Job drawing, mm, ordinate dimensions from the low corner. One solid piece. A direction names the side the tool comes from. Coordinates: 2 decimals unless noted, no trailing zeros. Order: outer loops, then holes, each group sorted by start corner. A loop starts at its lowest first (then second) coordinate and runs counter-clockwise, first axis right, second up. Notation, with made-up numbers: (82, 22) - (135, 22) arc R18 ccw to (135, 42) - close; hole circle Ø10 at (-24.75, 49.5). An arc over 180 degrees is marked (long way). Return JSON: item names as keys, results as strings.
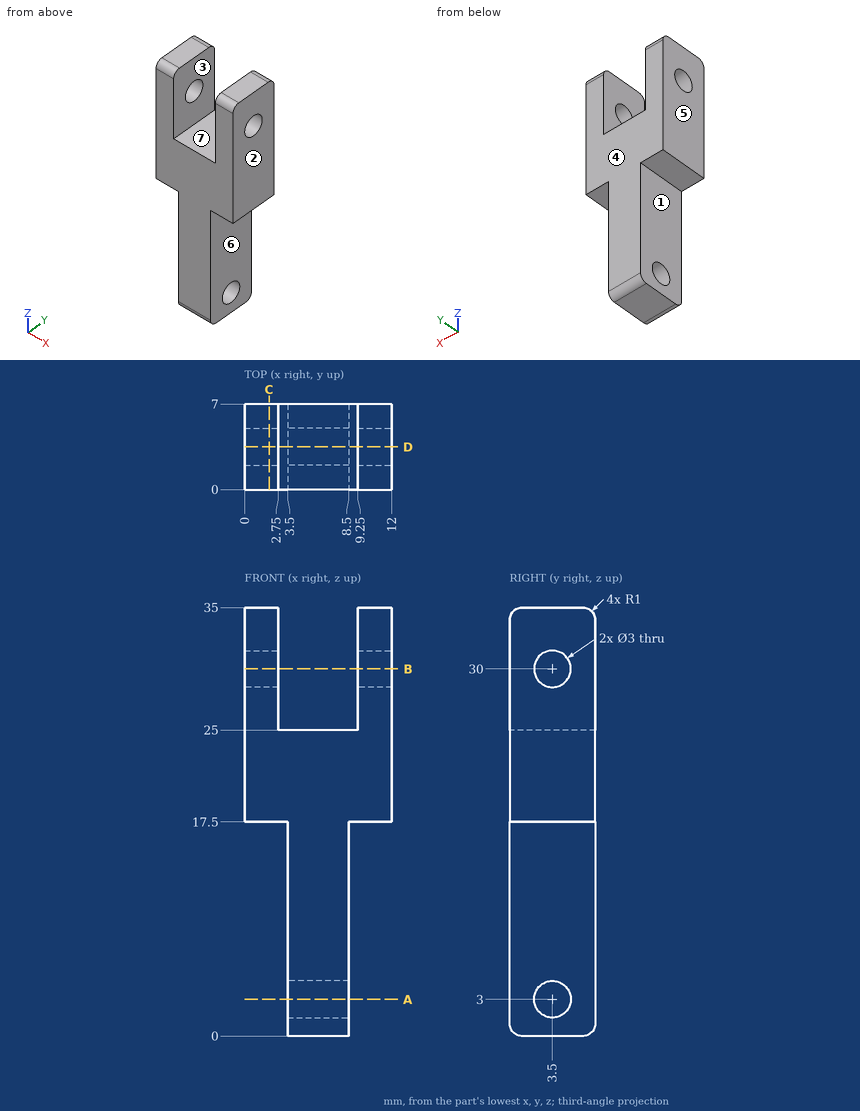
1. Cut at B-B on z = 30. Give the cut face in (x, y).
Check values:
{"outline": "(0, 0) - (2.75, 0) - (2.75, 2) - (0, 2) - close; (0, 5) - (2.75, 5) - (2.75, 7) - (0, 7) - close; (9.25, 0) - (12, 0) - (12, 2) - (9.25, 2) - close; (9.25, 5) - (12, 5) - (12, 7) - (9.25, 7) - close"}
2. Mould opens along X. For the marked faces 4, 5, 6 and 7 say: pulls with the +X half, pulls with the -X half, needs draft (parallel to the pull), parting line crosses it, or undercut.
Check values:
{"face 4": "needs draft", "face 5": "pulls with the -X half", "face 6": "pulls with the +X half", "face 7": "undercut"}
3. Tool access for the marked faces 1, 2 and 3: list every direction of +Z, -Z, +X, -X, +Y, -Y with a clear straight run to the whole face (end or side of a thin tool).
Check values:
{"face 1": "-Z, -X, +Y, -Y", "face 2": "+Z, -Z, +X, +Y, -Y", "face 3": "+Z, +Y, -Y"}
4. Drop flat-ended pins along their axis: pin 1 (3 mm diameter, centred on y = 2, z = 6.5, fed in from +X); pin 2 (1.8 mm diameter, centred on y = 3.5, z = 30, fed in from -X); pin 3 (3 mm diameter, centred on x = 1, y = 4.5, fed in from -Z); pin 4 (1 mm diameter, centred on y = 5, z = 12, fed in from -X). Give the stop position or say it passes through.
Check values:
{"pin 1": "x = 8.5", "pin 2": "through", "pin 3": "z = 17.5", "pin 4": "x = 3.5"}
5. Cut at D-D on y = 3.5. Give the cut face in (x, z), plus the area to 3 significant figures.
Check values:
{"outline": "(0, 17.5) - (3.5, 17.5) - (3.5, 4.5) - (8.5, 4.5) - (8.5, 17.5) - (12, 17.5) - (12, 28.5) - (9.25, 28.5) - (9.25, 25) - (2.75, 25) - (2.75, 28.5) - (0, 28.5) - close; (0, 31.5) - (2.75, 31.5) - (2.75, 35) - (0, 35) - close; (3.5, 0) - (8.5, 0) - (8.5, 1.5) - (3.5, 1.5) - close; (9.25, 31.5) - (12, 31.5) - (12, 35) - (9.25, 35) - close", "area": "201 mm²"}
6. Cut at C-C on x = 2. Give the cut face in (y, z).
Check values:
{"outline": "(0, 17.5) - (7, 17.5) - (7, 34) arc R1 ccw to (6, 35) - (1, 35) arc R1 ccw to (0, 34) - close; hole circle Ø3 at (3.5, 30)"}
7. Probe L1, parallel to X at y = 4.25, z = 27.5; L2, parallel to Y at x = 6.6, z = 3; L3, parallel to X at y = 1, z = 10.5. List the from-to ranges inside material, lowest first.
Check values:
{"L1": "0 to 2.75, 9.25 to 12", "L2": "0 to 2, 5 to 7", "L3": "3.5 to 8.5"}
8. Cut at A-A on z = 3. Give the cut face in (x, y), plus the area to 3 significant figures.
Check values:
{"outline": "(3.5, 0) - (8.5, 0) - (8.5, 2) - (3.5, 2) - close; (3.5, 5) - (8.5, 5) - (8.5, 7) - (3.5, 7) - close", "area": "20.0 mm²"}
